Design review of the part shown in the three views and the two pictorial views. Dimensions are in mm from the part's minimum x, y and z. Coordinates: 2 decimals unless noted, no trailing zeros. Loops run counter-clockwise (first coordinate to the right, second up) from the corner with the lowest first, then second, coordinate; pieces in that order, holes last. Notation, with made-up numbers: M 25.25,81.5 L 39.25,81.5 A18 ccw 39.25,88.5 Z; hole C 54,24 d5. An arc over 180 degrees is marked long. Put each result on its own line as item: value. Start each with the question number.
(1) Clearance check with flat-ended pins moving along their axes: pin 1 (8 mm diameter, centred on y = 160, z = 23.5, fed in from -X); pin 2 (3 mm diameter, centred on x = 3.5, z = 12, fed in from -Y); pin 3 (1.9 mm diameter, centred on x = 2.5, y = 212.5, fed in from -Z). State where each tip first meets the part, or that it passes through.
(2) Take a section at A-A, the plane y = 153. Give the boundary of the cut face in (x, z).
(3) For probe 1 along Z at (x, y) = (2, 163.5); probe 2 along Y at (x, z) = (1, 53.5), list the stretches that pass through material, from the lowest coordinate up. Write a range as [from, to].
(4) Take a section at B-B, the plane x = 3.25. Give the boundary of the cut face in (y, z), then the cut area to 3 significant figures.
(5) Take a section at C-C, the plane z = 61. Give the boundary of the cut face in (x, y), then the cut area to 3 significant figures.
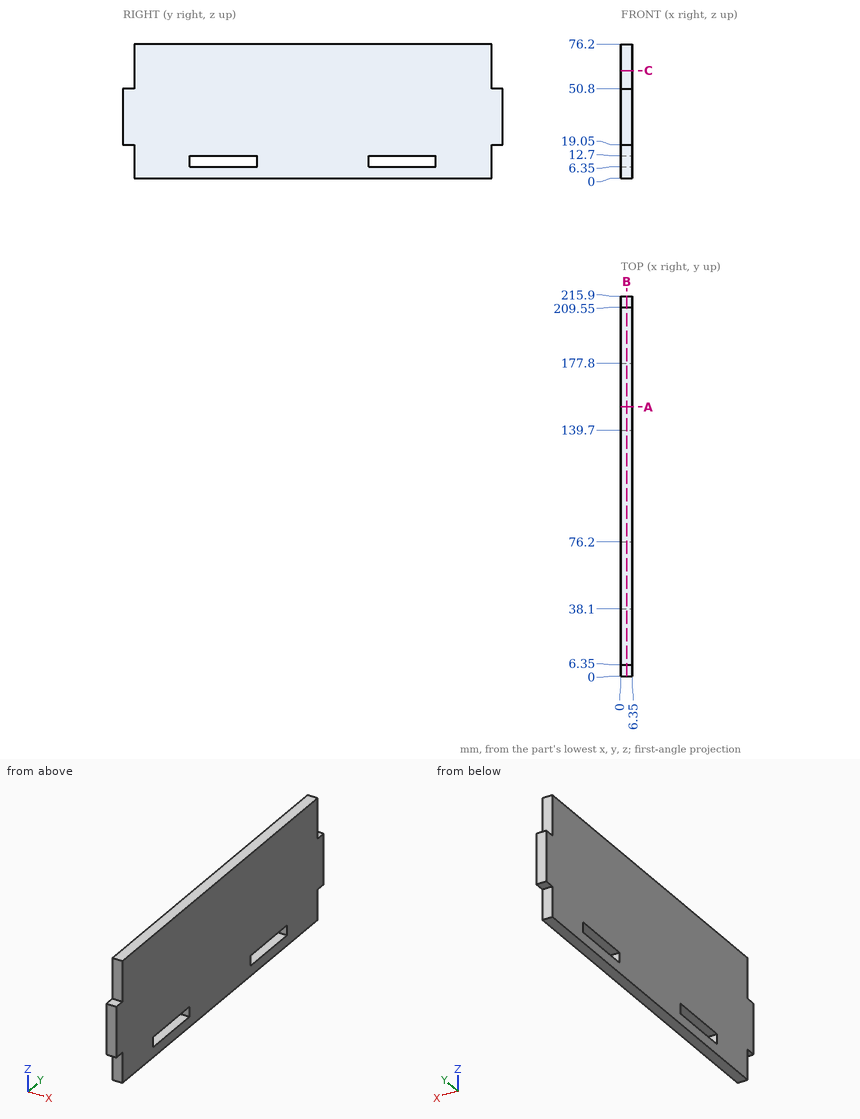
Computed values:
1. pin 1: stops at x = 0
1. pin 2: stops at y = 6.35
1. pin 3: stops at z = 19.05
2. outline: M 0,0 L 6.35,0 L 6.35,6.35 L 0,6.35 Z; M 0,12.7 L 6.35,12.7 L 6.35,76.2 L 0,76.2 Z
3. probe 1: z = [0, 6.35], [12.7, 76.2]
3. probe 2: y = [6.35, 209.55]
4. outline: M 0,19.05 L 6.35,19.05 L 6.35,0 L 209.55,0 L 209.55,19.05 L 215.9,19.05 L 215.9,50.8 L 209.55,50.8 L 209.55,76.2 L 6.35,76.2 L 6.35,50.8 L 0,50.8 Z; hole M 38.1,6.35 L 76.2,6.35 L 76.2,12.7 L 38.1,12.7 Z; hole M 139.7,6.35 L 177.8,6.35 L 177.8,12.7 L 139.7,12.7 Z
4. area: 15,400 mm^2
5. outline: M 0,6.35 L 6.35,6.35 L 6.35,209.55 L 0,209.55 Z
5. area: 1,290 mm^2
